from build123d import *

# Parameters (mm, degrees)
BOSS_EXTRUDE1_DEPTH = 13
CUT_EXTRUDE1_DEPTH  = 8.4
BOSS_EXTRUDE3_START = 5.7
BOSS_EXTRUDE3_DEPTH = 3
FILLET1_R           = 1.5
DRAFT2_ANGLE        = 3
FILLET2_R           = 3
FILLET3_R           = 2


with BuildPart() as part:
    # Sketch1 → Boss-Extrude1 (new body)
    with BuildSketch(Plane(origin=(0, 0, 0), x_dir=(1, 0, 0), z_dir=(0, 1, 0))):
        with BuildLine():
            Line((0, 0), (37.5, 0))
            ThreePointArc((37.5, 0), (50, 12.5), (37.5, 25))
            Line((37.5, 25), (0, 25))
            Line((0, 25), (0, 0))
        make_face()
    extrude(amount=BOSS_EXTRUDE1_DEPTH)

    # Sketch2 → Cut-Extrude1 (cut)
    with BuildSketch(Plane(origin=(0, 13, 0), x_dir=(1, 0, 0), z_dir=(0, 1, 0))):
        with BuildLine():
            Line((24.325, 19.675), (0, 19.675))
            Line((0, 19.675), (0, 5.325))
            Line((0, 5.325), (24.325, 5.325))
            ThreePointArc((24.325, 5.325), (31.5, 12.5), (24.325, 19.675))
        make_face()
    extrude(amount=-CUT_EXTRUDE1_DEPTH, mode=Mode.SUBTRACT)

    # Sketch3 → Boss-Extrude3 (add)
    with BuildSketch(Plane(origin=(0, 4.6, 0), x_dir=(1, 0, 0), z_dir=(0, 1, 0)).offset(BOSS_EXTRUDE3_START)):
        with BuildLine():
            Line((4, 5.325), (24.325, 5.325))
            ThreePointArc((24.325, 5.325), (26.969924385, 5.83029236), (29.242316341, 7.275))
            Line((29.242316341, 7.275), (4, 7.275))
            Line((4, 7.275), (4, 5.325))
        make_face()
        with BuildLine():
            Line((4, 19.675), (24.325, 19.675))
            ThreePointArc((24.325, 19.675), (26.969924385, 19.16970764), (29.242316341, 17.725))
            Line((29.242316341, 17.725), (4, 17.725))
            Line((4, 17.725), (4, 19.675))
        make_face()
    extrude(amount=-BOSS_EXTRUDE3_DEPTH)

    # Fillet1
    fillet1_edges = [part.edges().sort_by_distance(p)[0] for p in [
        (4, 7.3, -6.3),
        (4, 10.3, -6.3),
        (4, 7.3, -18.7),
        (4, 10.3, -18.7),
    ]]
    fillet(fillet1_edges, radius=FILLET1_R - 0.0001)  # a hair under: the kernel refuses the full size

    # Draft2
    draft2_faces = [part.faces().sort_by_distance(p)[0] for p in [
        (18.75, 6.5, -25),
        (50, 6.5, -12.5),
        (18.75, 6.5, 0),
    ]]
    draft(draft2_faces, Plane(origin=(37.5, 13, -12.5), x_dir=(0, 0, 1), z_dir=(0, 1, 0)), DRAFT2_ANGLE)

    # Fillet2
    fillet2_edges = [part.edges().sort_by_distance(p)[0] for p in [
        (0, 13, -2.6625),
        (0, 13, -22.3375),
    ]]
    fillet(fillet2_edges, radius=FILLET2_R)

    # Fillet3
    fillet3_edges = [part.edges().sort_by_distance(p)[0] for p in [
        (50, 13, -12.5),
        (20.25, 13, -25),
        (20.25, 13, 0),
        (0, 5, -25.419262234),
        (0, 5, 0.419262234),
        (0.877952484, 12.120592922, -25.046087772),
        (0.877952484, 12.120592922, 0.046087772),
    ]]
    fillet(fillet3_edges, radius=FILLET3_R)


solid = part.part
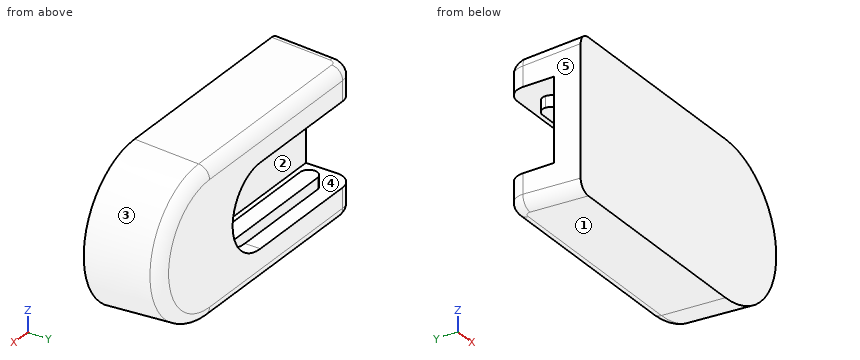
Geometry check sheet. Reference: the model listing, model coordinates, mm. Face numbers are marked on the shaded views. A direction names the side the tool comes from. Round coordinates to 2 decimals unless told otherwise and drop trailing zeros. Order: outer loops, then holes, each group sorted by start corner. A loop starts at its lowest first (then second) coordinate and runs counter-clockwise, first axis right, second up. Notation, with made-up numbers: M 44,-29 L 72,-29 A25 ccw 72,5 Z; hole C 28,12.25 d11. An arc over 180 degrees is marked long. Write each question's results on one line, items separated by ' | '. Start each with the question number.
1. Material ranges on L1, parallel to Z at x = 25, y = 10 (3 decimals); L2, parallel to Y at x = 26.5, z = -16; L3, parallel to Y at x = 26, z = -18.5, recorded low to high. Write a range as from..to.
2. Draft check along Y on the marked faces 3, 4 and 5. Enter one of: pulls with the +Y half, pulls with the -Y half, needs draft (parallel to the pull), parting line crosses it, or undercut.
3. Go/stop test with flat-tipped pins: P1, Ø2.5, axis at x = 6.5, y = 9.5, coming from the +Z side; P2, Ø3.5, axis at x = 13.5, y = 9, coming from the +Z side; P3, Ø1.5, axis at x = 13.5, y = 9.5, coming from the -Z side. Record where each tip stops, or that it passes through.
4. Cross-section at B-B on z = -12.5. Record the boundary of the cut face in (x, y), plus the area to 3 significant figures.
5. Cross-section at A-A on x = 8. Record the boundary of the cut face in (y, z) (3 decimals), plus the area to 3 significant figures.
6. Cross-section at C-C on x = 35. Record the boundary of the cut face in (y, z), plus the area to 3 significant figures.
7. Set-up check for the marked faces 1 and 2: record each of +Z, -Z, +X, -X, +Y, -Y from which the full face is reachable in a straight line by a thin tool's end or side.
Resolved:
1) L1: -25.157..-17.725, -7.275..0.157 | L2: 0..4.6 | L3: 0..4.6, 7.3..10.3
2) face 3: pulls with the +Y half | face 4: undercut | face 5: needs draft
3) P1: z = 0.25 | P2: z = 0.3 | P3: z = -25.22
4) outline: M 0,0 L 50.68,0 L 50.1,11.1 A2 ccw 48.1,13 L 31.5,13 L 31.5,4.6 L 0,4.6 Z | area: 389 mm2
5) outline: M 0,-25.681 L 11.105,-25.099 A2 ccw 13,-23.102 L 13,-19.675 L 10.3,-19.675 L 10.3,-17.725 L 7.3,-17.725 L 7.3,-19.675 L 4.6,-19.675 L 4.6,-5.325 L 7.3,-5.325 L 7.3,-7.275 L 10.3,-7.275 L 10.3,-5.325 L 13,-5.325 L 13,-1.898 A2 ccw 11.105,0.099 L 0,0.681 Z | area: 223 mm2
6) outline: M 0,-25.68 L 11.1,-25.1 A2 ccw 13,-23.1 L 13,-1.9 A2 ccw 11.1,0.1 L 0,0.68 Z | area: 332 mm2
7) face 1: -Z, +X, -X, +Y | face 2: -X
